```python
from build123d import *

# Parameters (mm, degrees)
EXTRUDE_2_DEPTH     = 60
SKETCH_3_R          = 1.5
CUT_EXTRUDE_1_DEPTH = 40
SKETCH_7_W          = 35
SKETCH_7_H          = 50
EXTRUDE_4_DEPTH     = 2
SKETCH_8_R          = 1.5
CUT_EXTRUDE_3_DEPTH = 12
FILLET_1_R          = 4


with BuildPart() as part:
    # 草图1 → 凸台-拉伸2 (new body)
    with BuildSketch(Plane.XY):
        Polygon((-29.5, 30), (-27.5, 30), (-27.5, 3), (27.5, 3), (27.5, 25), (29.5, 25), (29.5, -25), (27.5, -25), (27.5, -3), (-27.5, -3), (-27.5, -30), (-29.5, -30), align=None)
    extrude(amount=EXTRUDE_2_DEPTH)

    # 草图3 → 切除-拉伸1 (cut)
    with BuildSketch(Plane.ZY.offset(29.5)):
        with Locations(Location((51, 21, 0), (0, 0, 270))):
            Circle(SKETCH_3_R)
        with Locations(Location((51, -21, 0), (0, 0, 270))):
            Circle(SKETCH_3_R)
        with Locations(Location((9, 21, 0), (0, 0, 270))):
            Circle(SKETCH_3_R)
        with Locations(Location((9, -21, 0), (0, 0, 270))):
            Circle(SKETCH_3_R)
    extrude(amount=-CUT_EXTRUDE_1_DEPTH, mode=Mode.SUBTRACT)

    # 草图7 → 凸台-拉伸4 (add)
    with BuildSketch(Plane.ZY.offset(-27.5)):
        with Locations((42.5, 50)):
            Rectangle(SKETCH_7_W, SKETCH_7_H)
        with Locations((42.5, -50)):
            Rectangle(SKETCH_7_W, SKETCH_7_H)
    extrude(amount=-EXTRUDE_4_DEPTH)

    # 草图8 → 切除-拉伸3 (cut)
    with BuildSketch(Plane.ZY.offset(-27.5)):
        with Locations(Location((34.25, 70, 0), (0, 0, 270))):
            Circle(SKETCH_8_R)
        with Locations(Location((34.25, -70, 0), (0, 0, 270))):
            Circle(SKETCH_8_R)
    extrude(amount=-CUT_EXTRUDE_3_DEPTH, mode=Mode.SUBTRACT)

    # 圆角1
    fillet_1_edges = [part.edges().sort_by_distance(p)[0] for p in [
        (-28.5, 30, 0),
        (28.5, 25, 0),
        (28.5, -25, 0),
        (-28.5, -30, 0),
        (-28.5, 30, 60),
        (28.5, 25, 25),
        (28.5, 75, 25),
        (28.5, 75, 60),
        (28.5, -25, 25),
        (28.5, -75, 60),
        (28.5, -75, 25),
        (-28.5, -30, 60),
    ]]
    fillet(fillet_1_edges, radius=FILLET_1_R)


solid = part.part
```
Design review of the part built by this model. Coordinates are the model's own, in mm. A direction names the side the tool comes from. Coordinates: 2 decimals unless noted, no trailing zeros. Loops run counter-clockwise (first coordinate to the right, second up) from the corner with the lowest first, then second, coordinate; pieces in that order, holes last. Notation, with made-up numbers: (9.5, 77.25) - (52.5, 77.25) arc R12 ccw to (52.5, 86.25) - close; hole circle Ø8 at (42, 74). An arc over 180 degrees is marked (long way). Use CSV: the item, a comma, the result in double quotes. Start each with the question number.
1) Tool access review of faces 1 (the cylindrical face through (-28.51, -19.5, 9.07)), 2 (the cylindrical face through (-28.514, -28.797, 58.859)), 3 (the flat face through (27.5, -32, 36)): name each direction out of +Z, -Z, +X, -X, +Y, -Y from which nothing blocks a thin tool from reaching the whole face with its end or side.
2) Consider section D-D on y = 65. Write out the cut boundary in (x, z).
3) Consider section C-C on z = 43. Write out the cut boundary in (x, y).
4) Consider section A-A on z = 34.25. Write out the cut boundary in (x, y).
5) Consider section B-B on y = -11. Write out the cut boundary in (x, z), then the cut area to 3 significant figures.
6) Wall thickness on L1, parallel to Z at x = -28.6, y = -21; L2, parallel to X at y = 5, z = 37; L3, parallel to Y at x = -16, z = 4: over which ranges is each line inside the solid? List them lowest first. Write a range as from..to.
7) For pin 1 Ø1 at (x, y) = (28.5, 53) entering from -Z; pin 2 Ø1 at (x, z) = (28, 10) entering from -Y; pin 3 Ø1 at (x, z) = (-28.5, 37) entering from -Y, all flat-tipped, find the tip position at first contact; note any pin that passes through.
8) The part is to be moulded in two halves that separate along X. For faces 4 (the flat face through (29.5, 1, 36)), 5 (the cylindrical face through (28.514, 23.859, 1.203)), 6 (the flat face through (27.5, 32, 36)), say which applies: +X half, -X half, draft (parallel to the pull), parting line (faces both ways), or undercut.
Geometry says:
1,face 1,"-X"
1,face 2,"+Z, -X, -Y"
1,face 3,"+Z, -Z, -Y"
2,outline,"(27.5, 25) - (29.5, 25) - (29.5, 60) - (27.5, 60) - close"
3,outline,"(-29.5, -30) - (-27.5, -30) - (-27.5, -3) - (27.5, -3) - (27.5, -75) - (29.5, -75) - (29.5, 75) - (27.5, 75) - (27.5, 3) - (-27.5, 3) - (-27.5, 30) - (-29.5, 30) - close"
4,outline,"(-29.5, -30) - (-27.5, -30) - (-27.5, -3) - (27.5, -3) - (27.5, -68.5) - (29.5, -68.5) - (29.5, 68.5) - (27.5, 68.5) - (27.5, 3) - (-27.5, 3) - (-27.5, 30) - (-29.5, 30) - close; (27.5, -75) - (29.5, -75) - (29.5, -71.5) - (27.5, -71.5) - close; (27.5, 71.5) - (29.5, 71.5) - (29.5, 75) - (27.5, 75) - close"
5,outline,"(-29.5, 0) - (-27.5, 0) - (-27.5, 60) - (-29.5, 60) - close; (27.5, 0) - (29.5, 0) - (29.5, 60) - (27.5, 60) - close"
5,area,"240 mm^2"
6,L1,"0..7.5, 10.5..49.5, 52.5..60"
6,L2,"-29.5..-27.5, 27.5..29.5"
6,L3,"-3..3"
7,pin 1,"z = 25"
7,pin 2,"y = -25"
7,pin 3,"y = -30"
8,face 4,"+X half"
8,face 5,"draft"
8,face 6,"undercut"
